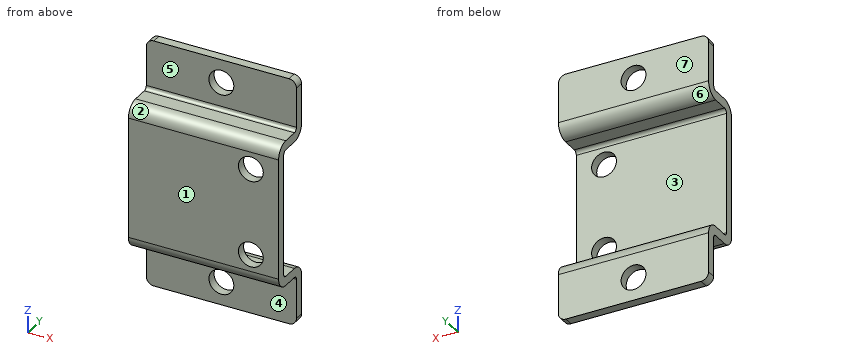
```python
from build123d import *

# Parameters (mm, degrees)
F1_DEPTH = 13
F2_R     = 2.15
F3_DEPTH = 7.2010003069
F4_R     = 1.3


# Not quite as in the source:
# - ends of sketch curves that miss each other by under 0.0002 mm in the source are joined


with BuildPart() as f1:
    # F0 (on Right) → F1 (new body, symmetric)
    with BuildSketch(Plane.YZ):
        with BuildLine():
            Line((-3.3650011141, 32.6000002232), (-0.6352006896, 32.6000002232))
            ThreePointArc((-0.6352006896, 32.6000002232), (0.9453246879, 33.2546752703), (1.5999997349, 34.8352006478))
            Line((1.5999997349, 34.8352006478), (1.5999997349, 41.7300015539))
            Line((1.5999997349, 41.7300015539), (1.5999997349, 43.0000009998))
            Line((1.5999997349, 43.0000009998), (0, 43))
            Line((0, 43), (0, 41.7300015539))
            Line((0, 41.7300015539), (0, 34.8350006809))
            ThreePointArc((0, 34.8350006809), (-0.1859871128, 34.3859880708), (-0.634999723, 34.200000958))
            Line((-0.634999723, 34.200000958), (-3.3648001474, 34.200000958))
            ThreePointArc((-3.3648001474, 34.200000958), (-4.945325525, 33.5453259109), (-5.600000572, 31.9648005334))
            Line((-5.600000572, 31.9648005334), (-5.600000572, 11.0352004664))
            ThreePointArc((-5.600000572, 11.0352004664), (-4.945325525, 9.4546750889), (-3.3648001474, 8.8000000419))
            Line((-3.3648001474, 8.8000000419), (-0.634999723, 8.8000000419))
            ThreePointArc((-0.634999723, 8.8000000419), (-0.1859871128, 8.6140129291), (0, 8.1650003189))
            Line((0, 8.1650003189), (0, 1.2700004457))
            Line((0, 1.2700004457), (0, 0))
            Line((0, 0), (1.5999997349, 0))
            Line((1.5999997349, 0), (1.5999997349, 1.2700004457))
            Line((1.5999997349, 1.2700004457), (1.5999997349, 8.1648003521))
            ThreePointArc((1.5999997349, 8.1648003521), (0.9453246879, 9.7453257296), (-0.6352006896, 10.4000007766))
            Line((-0.6352006896, 10.4000007766), (-3.3650011141, 10.4000007766))
            ThreePointArc((-3.3650011141, 10.4000007766), (-3.8140137243, 10.5859878894), (-4.0000008371, 11.0350004996))
            Line((-4.0000008371, 11.0350004996), (-4.0000008371, 31.9650005003))
            ThreePointArc((-4.0000008371, 31.9650005003), (-3.8140137243, 32.4140131104), (-3.3650011141, 32.6000002232))
        make_face()
    extrude(amount=F1_DEPTH, both=True)

    # F2 (on face) → F3 (cut, through all)
    with BuildSketch(Plane.XZ.offset(5.600000572)):
        with Locations((0, 4)):
            Circle(F2_R)
        with Locations((0, 39)):
            Circle(F2_R)
        with Locations((8.1994, 29)):
            Circle(F2_R)
        with Locations((8.1994, 14)):
            Circle(F2_R)
    extrude(amount=-F3_DEPTH, mode=Mode.SUBTRACT)

    # F4
    f4_edges = [f1.edges().sort_by_distance(p)[0] for p in [
        (-13, 0.8, 43),
        (-13, 0.8, 0),
        (13, 0.8, 0),
        (13, 0.8, 43),
    ]]
    fillet(f4_edges, radius=F4_R)


solid = f1.part
```
Work out the finished part from the listing and answer in its coordinate system (mm). Face numbers are marked on the shaded views. A direction names the side the tool comes from. Round coordinates to 2 decimals unless told otherwise and drop trailing zeros. Write each loop counter-clockwise with the first axis right and the second up, starting at its lowest first coordinate (ties: lowest second). Pieces come first, ordered by that corner, then holes.
1) Consider probe 1 along Z at (x, y) = (7, -1.5); probe 2 along Y at (x, z) = (-10.75, 14); probe 3 along Z at (x, y) = (0, 1.2). Determine where each line is inside the solid, lowest interval first.
2) A cutting plane is placed at C-C on x = 3.25. Determine the outline of the cut face in (y, z) (3 decimals).
3) A cutting plane is placed at B-B on x = 0. Determine the outline of the cut face in (y, z) (3 decimals).
4) Determine the mould class of the marked faces 1, 2 and 3 for opening direction Z: pulls with the +Z half, pulls with the -Z half, needs draft (parallel to the pull), parting line crosses it, or undercut.
5) Flat-ended cylindrical pins translate along their axes: P1, Ø0.8, axis at x = 5.5, y = -2.5, coming from the +Z side; P2, Ø2.5, axis at x = 3, z = 3.5, coming from the -Y side; P3, Ø3, axis at x = 0, y = -2, coming from the -Z side. Find the tip coordinate at first contact, or state that the pin passes through.
6) A cutting plane is placed at A-A on z = 14. Determine the outline of the cut face in (x, y), and give its area (3 significant figures).
7) A cutting plane is placed at D-D on y = -4.75. Determine the outline of the cut face in (x, z).
8) Which of the six approach directions +Z, -Z, +X, -X, +Y, -Y give full straight-line access (tool end or side, diameter ignored) to the marked faces 4, 5, 6 and 7?
Entries:
1. probe 1: z = 8.8 to 10.4, 32.6 to 34.2
1. probe 2: y = -5.6 to -4
1. probe 3: z = 0 to 1.85, 6.15 to 9.44, 33.56 to 36.85, 41.15 to 43
2. outline: (-5.6, 11.035) arc R2.235 ccw to (-3.365, 8.8) - (-0.635, 8.8) arc R0.635 cw to (0, 8.165) - (0, 0) - (1.6, 0) - (1.6, 8.165) arc R2.235 ccw to (-0.635, 10.4) - (-3.365, 10.4) arc R0.635 cw to (-4, 11.035) - (-4, 31.965) arc R0.635 cw to (-3.365, 32.6) - (-0.635, 32.6) arc R2.235 ccw to (1.6, 34.835) - (1.6, 43) - (0, 43) - (0, 34.835) arc R0.635 cw to (-0.635, 34.2) - (-3.365, 34.2) arc R2.235 ccw to (-5.6, 31.965) - close
3. outline: (-5.6, 11.035) arc R2.235 ccw to (-3.365, 8.8) - (-0.635, 8.8) arc R0.635 cw to (0, 8.165) - (0, 6.15) - (1.6, 6.15) - (1.6, 8.165) arc R2.235 ccw to (-0.635, 10.4) - (-3.365, 10.4) arc R0.635 cw to (-4, 11.035) - (-4, 31.965) arc R0.635 cw to (-3.365, 32.6) - (-0.635, 32.6) arc R2.235 ccw to (1.6, 34.835) - (1.6, 36.85) - (0, 36.85) - (0, 34.835) arc R0.635 cw to (-0.635, 34.2) - (-3.365, 34.2) arc R2.235 ccw to (-5.6, 31.965) - close; (0, 0) - (1.6, 0) - (1.6, 1.85) - (0, 1.85) - close; (0, 41.15) - (1.6, 41.15) - (1.6, 43) - (0, 43) - close
4. face 1: needs draft
4. face 2: pulls with the +Z half
4. face 3: undercut
5. P1: stops at z = 34.2
5. P2: stops at y = 0
5. P3: stops at z = 8.79
6. outline: (-13, -5.6) - (6.05, -5.6) - (6.05, -4) - (-13, -4) - close; (10.35, -5.6) - (13, -5.6) - (13, -4) - (10.35, -4) - close
6. area: 34.7 mm2
7. outline: (-13, 9.28) - (13, 9.28) - (13, 33.72) - (-13, 33.72) - close; hole circle Ø4.3 at (8.2, 14); hole circle Ø4.3 at (8.2, 29)
8. face 4: -Z, +X, -X, -Y
8. face 5: +Z, +X, -X, -Y
8. face 6: +X, -X, +Y
8. face 7: +Z, -Z, +X, -X, +Y
